```python
from build123d import *

# Parameters (mm, degrees)
SKETCH1_W           = 79.7
SKETCH1_H           = 20
SKETCH1_R           = 3.25
BOSS_EXTRUDE1_DEPTH = 5
SKETCH2_W           = 8
SKETCH2_H           = 5
BOSS_EXTRUDE2_DEPTH = 10
BOSS_EXTRUDE3_DEPTH = 5
SKETCH3_6_R         = 2.5
CUT_EXTRUDE2_DEPTH  = 84.295197941


with BuildPart() as part:
    # Sketch1 → Boss-Extrude1 (new body)
    with BuildSketch(Plane(origin=(0, 0, 0), x_dir=(0, 0, -1), z_dir=(1, 0, 0))):
        with Locations((-39.85, 10)):
            Rectangle(SKETCH1_W, SKETCH1_H)
        with Locations((-29.9, 10)):
            Circle(SKETCH1_R, mode=Mode.SUBTRACT)
        with Locations((-49.8, 10)):
            Circle(SKETCH1_R, mode=Mode.SUBTRACT)
        with Locations((-69.7, 10)):
            Circle(SKETCH1_R, mode=Mode.SUBTRACT)
        with Locations((-10, 10)):
            Circle(SKETCH1_R, mode=Mode.SUBTRACT)
    extrude(amount=BOSS_EXTRUDE1_DEPTH)

    # Sketch2 → Boss-Extrude2 (add)
    with BuildSketch(Plane(origin=(5, 0, 0), x_dir=(0, 0, -1), z_dir=(1, 0, 0))):
        with Locations((-19.925, 2.5)):
            Rectangle(SKETCH2_W, SKETCH2_H)
        with Locations((-59.775, 2.5)):
            Rectangle(SKETCH2_W, SKETCH2_H)
    extrude(amount=BOSS_EXTRUDE2_DEPTH)

    # Sketch3 → Boss-Extrude3 (add)
    with BuildSketch(Plane(origin=(0, 5, 0), x_dir=(1, 0, 0), z_dir=(0, 1, 0))):
        with BuildLine():
            Line((15, -55.775), (15, -63.775))
            ThreePointArc((15, -63.775), (19, -59.775), (15, -55.775))
        make_face()
    boss_extrude3 = extrude(amount=-BOSS_EXTRUDE3_DEPTH)

    # Sketch3_6 → Cut-Extrude2 (cut, through all)
    with BuildSketch(Plane(origin=(0, 5, 0), x_dir=(1, 0, 0), z_dir=(0, 1, 0))):
        with Locations(Location((15, -59.775, 0), (0, 0, 270))):
            Circle(SKETCH3_6_R)
    cut_extrude2 = extrude(amount=-CUT_EXTRUDE2_DEPTH, mode=Mode.SUBTRACT)

    # Mirror1: Boss-Extrude3, Cut-Extrude2 across plane
    add(boss_extrude3.mirror(Plane.XY.offset(39.85)))
    add(cut_extrude2.mirror(Plane.XY.offset(39.85)), mode=Mode.SUBTRACT)


solid = part.part
```
Geometry check sheet. Reference: the model listing, model coordinates, mm. A direction names the side the tool comes from. Coordinates: 2 decimals unless noted, no trailing zeros. Order: outer loops, then holes, each group sorted by start corner. A loop starts at its lowest first (then second) coordinate and runs counter-clockwise, first axis right, second up. Notation, with made-up numbers: (88.5, 22.5) - (131.5, 22.5) arc R24 ccw to (131.5, 34.5) - close; hole circle Ø4 at (-35, 77). An arc over 180 degrees is marked (long way). Use one line per item in the form item = value.
1. Scan lines: line 1 (Y direction, x = 3.6, z = 49.8); line 2 (X direction, y = 4, z = 29.5). Record each from-to range of solid material in increasing order.
Here are the results:
line_1 = 0 to 6.75, 13.25 to 20
line_2 = 0 to 5
2. Section check B-B (x = 16.5). Record the boundary of the cut face in (y, z) (3 decimals).
Here are the results:
outline = (0, 16.217) - (5, 16.217) - (5, 17.925) - (0, 17.925) - close; (0, 21.925) - (5, 21.925) - (5, 23.633) - (0, 23.633) - close; (0, 56.067) - (5, 56.067) - (5, 57.775) - (0, 57.775) - close; (0, 61.775) - (5, 61.775) - (5, 63.483) - (0, 63.483) - close
3. Access from +Z, -Z, +X, -X, +Y, -Y to the whole of each face (thin tool, end or side, straight path). Record for faces 1 (the face through (10, 2, 63.775)), 2 (the face through (10, 2, 23.925)), 3 (the face through (10, 5, 20)), 4 (the face through (10, 2, 15.925)).
Here are the results:
face_1 = +Z, +X, +Y, -Y
face_2 = +X, +Y, -Y
face_3 = +Z, -Z, +X, +Y
face_4 = -Z, +X, +Y, -Y
4. Section check D-D (y = 11). Record the boundary of the cut face in (x, z).
Here are the results:
outline = (0, 0) - (5, 0) - (5, 6.91) - (0, 6.91) - close; (0, 13.09) - (5, 13.09) - (5, 26.81) - (0, 26.81) - close; (0, 32.99) - (5, 32.99) - (5, 46.71) - (0, 46.71) - close; (0, 52.89) - (5, 52.89) - (5, 66.61) - (0, 66.61) - close; (0, 72.79) - (5, 72.79) - (5, 79.7) - (0, 79.7) - close
5. Section check C-C (z = 49.8). Record the boundary of the cut face in (x, y), then the cut area to 3 significant figures.
Here are the results:
outline = (0, 0) - (5, 0) - (5, 6.75) - (0, 6.75) - close; (0, 13.25) - (5, 13.25) - (5, 20) - (0, 20) - close
area = 67.5 mm²
6. Draft check along X on faces 5 (the face through (19, 3, 20)), 6 (the face through (2.465, 12.197, 12.395)), 7 (the face through (12.56, 2.54, 59.23)). Enter one of: pulls with the +X half, pulls with the -X half, needs draft (parallel to the pull), parting line crosses it, or undercut.
Here are the results:
face_5 = pulls with the +X half
face_6 = needs draft
face_7 = undercut
7. Gauge pin test, flat ends, axial feed: pin 1 (6 mm diameter, centred on x = 13.5, y = 7.5, fed in from +Z) (3 decimals); pin 2 (1.5 mm diameter, centred on x = 12, y = 2.5, fed in from -Z) (3 decimals); pin 3 (6 mm diameter, centred on x = 12.5, z = 24.5, fed in from +Y). Record the tip position at first contact, or that the pin passes through.
Here are the results:
pin_1 = 63.775
pin_2 = 15.925
pin_3 = 5
8. Section check A-A (y = 1.5). Record the boundary of the cut face in (x, z) (3 decimals).
Here are the results:
outline = (0, 0) - (5, 0) - (5, 15.925) - (15, 15.925) arc R4 ccw to (15, 23.925) - (5, 23.925) - (5, 55.775) - (15, 55.775) arc R4 ccw to (15, 63.775) - (5, 63.775) - (5, 79.7) - (0, 79.7) - close; hole circle Ø5 at (15, 19.925); hole circle Ø5 at (15, 59.775)
